from build123d import *

# Parameters (mm, degrees)
PAD_DEPTH       = 4
PAD001_DEPTH    = 2
SKETCH004_R     = 4.1
POCKET002_DEPTH = 32.7030832918
SKETCH001_R     = 2.1
POCKET_DEPTH    = 5
SKETCH002_R     = 1.15
POCKET001_DEPTH = 33.4827417793
CHAMFER_SIZE    = 0.99


with BuildPart() as part:
    # Sketch → Pad (new body, symmetric)
    with BuildSketch(Plane.XZ):
        with BuildLine():
            Line((-1.1974254129, -3.2898992834), (-12.1420699993, -33.3600631485))
            ThreePointArc((-12.1420699993, -33.3600631485), (-11.5443975218, -34.6417759126), (-10.2626847577, -34.0441034352))
            Line((-10.2626847577, -34.0441034352), (0.6819598287, -3.97393957))
            ThreePointArc((3.501037691, -2), (1.780308382, -2.5425438671), (0.6819598287, -3.97393957))
            Line((3.501037691, -2), (22, -2))
            ThreePointArc((22, -2), (23, -1), (22, 0))
            Line((3.501037691, 0), (22, 0))
            ThreePointArc((3.501037691, 0), (0.6331555093, -0.9042397786), (-1.1974254129, -3.2898992834))
        make_face()
    extrude(amount=PAD_DEPTH, both=True)

    # Sketch003 → Pad001 (join)
    with BuildSketch(Plane.XZ.offset(-4)):
        with BuildLine():
            Line((-1.1974254129, -3.2898992834), (-12.1420699993, -33.3600631485))
            Line((-12.1420699993, -33.3600631485), (-10.2626847577, -34.0441034352))
            ThreePointArc((-7.9645514284, -32.1157406061), (-9.3719697244, -32.7720305358), (-10.2626847577, -34.0441034352))
            ThreePointArc((-7.9645514284, -32.1157406061), (-6.5571331323, -31.4594506764), (-5.666418099, -30.1873777771))
            Line((-5.666418099, -30.1873777771), (2.3036122782, -8.2898992834))
            ThreePointArc((7.0020753821, -5), (4.1341932003, -5.9042397786), (2.3036122782, -8.2898992834))
            Line((9.8038475773, -5), (7.0020753821, -5))
            ThreePointArc((9.8038475773, -5), (11.3038475773, -4.5980762114), (12.4019237887, -3.5))
            ThreePointArc((15, -2), (13.5, -2.4019237887), (12.4019237887, -3.5))
            Line((15, 0), (15, -2))
            Line((3.501037691, 0), (15, 0))
            ThreePointArc((3.501037691, 0), (0.6331555093, -0.9042397786), (-1.1974254129, -3.2898992834))
        make_face()
    extrude(amount=PAD001_DEPTH)

    # Sketch004 → Pocket002 (cut, through all)
    with BuildSketch(Plane.XY.offset(-2)):
        with Locations((18, 0)):
            Circle(SKETCH004_R)
    extrude(amount=-POCKET002_DEPTH, mode=Mode.SUBTRACT)

    # Sketch001 → Pocket (cut)
    with BuildSketch(Plane.XY):
        with Locations((18, 0)):
            Circle(SKETCH001_R)
    extrude(amount=-POCKET_DEPTH, mode=Mode.SUBTRACT)

    # Sketch002 (on Face2 of Pocket) → Pocket001 (cut, through all)
    with BuildSketch(Plane(origin=(0, 0, 0), x_dir=(-0.3420201433, 0, -0.9396926208), z_dir=(-0.9396926208, 0, 0.3420201433))):
        with Locations((4, 0)):
            Circle(SKETCH002_R)
        with Locations((34, 0)):
            Circle(SKETCH002_R)
    extrude(amount=-POCKET001_DEPTH, mode=Mode.SUBTRACT)

    # Chamfer
    chamfer_edges = [part.edges().sort_by_distance(p)[0] for p in [
        (15.9, 0, -2),
    ]]
    chamfer(chamfer_edges, length=CHAMFER_SIZE)


solid = part.part
Design review of the part built by this model. Coordinates are the model's own, in mm. A direction names the side the tool comes from. Round coordinates to 2 decimals unless told otherwise and drop trailing zeros. Order: outer loops, then holes, each group sorted by start corner. A loop starts at its lowest first (then second) coordinate and runs counter-clockwise, first axis right, second up. Notation, with made-up numbers: M 3,84.5 L 51,84.5 A22 ccw 51,114.5 Z; hole C 22,-37 d1. An arc over 180 degrees is marked long. Answer as CSV lines item,"result". Start each with the question number.
1) Wall thickness on line 1 along Y through (x, z) = (18, -0.5); line 2 along Z through (x, y) = (15, -2.5); line 3 along Y through (x, z) = (10.5, -4.5): over which ranges is each line inside the solid? List them lowest first. Write a range as [from, to].
2) Tool access review of faces 1 (the face through (-1, 2, -14)), 2 (the face through (20.003, 0.631, -0.498)), 3 (the face through (8, 3, -5)): name each direction out of +Z, -Z, +X, -X, +Y, -Y from which nothing blocks a thin tool from reaching the whole face with its end or side.
3) Add section A-A (x = 18). Give the boundary of the cut face in (y, z).
4) The part is to be moulded in two halves that separate along Z. For faces 4 (the face through (-10.309, -0.051, -31.207)), 5 (the face through (1.8, -1.04, -2.53)), 6 (the face through (0, 4, -13)), 7 (the face through (-0.78, -0.35, -5.14)), say which applies: +Z half, -Z half, draft (parallel to the pull), parting line (faces both ways), or undercut.
5) Add section D-D (z = -19). Give the boundary of the cut face in (x, y).
6) For pin 1 Ø7.5 at (x, z) = (1.5, -23) entering from -Y; pin 2 Ø1 at (y, z) = (2.5, -27) entering from -X; pin 3 Ø2 at (y, z) = (2, -30.5) entering from -X; pin 4 Ø2 at (x, y) = (8.5, -2) entering from +Z, all flat-tipped, find the tip position at first contact; note any pin that passes through.
7) Add section C-C (z = -1.5). Give the boundary of the cut face in (x, y).
8) Add section B-B (y = 0). Give the boundary of the cut face in (x, z).
Resolved:
1,line 1,"[-4, -2.1], [2.1, 4]"
1,line 2,"[-2, 0]"
1,line 3,"[2, 4]"
2,face 1,"-Z, +X, -Y"
2,face 2,"+Z, -Z"
2,face 3,"-Z, +X, +Y, -Y"
3,outline,"M -4,-2 L -3.09,-2 L -2.1,-1.01 L -2.1,0 L -4,0 Z; M 2.1,-1.01 L 3.09,-2 L 4,-2 L 4,0 L 2.1,0 Z"
4,face 4,"undercut"
4,face 5,"-Z half"
4,face 6,"draft"
4,face 7,"undercut"
5,outline,"M -6.92,-4 L -4.79,-4 L -4.79,2 L -1.59,2 L -1.59,4 L -6.92,4 Z"
6,pin 1,"through"
6,pin 2,"x = -10.01"
6,pin 3,"x = -11.47"
6,pin 4,"z = 0"
7,outline,"M -0.07,-4 L 22.87,-4 L 22.87,4 L -0.07,4 Z; hole C 18,0 d5.18"
8,outline,"M -12.14,-33.36 A1 ccw -10.26,-34.04 L -10.14,-33.71 L -12.02,-33.03 Z; M -11.24,-30.87 L -9.36,-31.55 L 0.12,-5.52 L -1.76,-4.84 Z; M -0.93,-2.69 L 0.97,-3.39 A3 cw 3.5,-2 L 14.91,-2 L 15.9,-1.01 L 15.9,0 L 3.5,0 A5 ccw Z; M 20.1,-1.01 L 21.09,-2 L 22,-2 A1 ccw 22,0 L 20.1,0 Z"
